from build123d import *

# Parameters (mm, degrees)
SKETCH2_R           = 2.5
BOSS_EXTRUDE1_DEPTH = 10
BOSS_EXTRUDE2_DEPTH = 2
FILLET1_R           = 2


with BuildPart() as part:
    # Sketch2 → Boss-Extrude1 (new body)
    with BuildSketch(Plane(origin=(0, 0, 0), x_dir=(1, 0, 0), z_dir=(0, 1, 0))):
        with BuildLine():
            Line((-68.25, 22.5), (-68.25, -7.5))
            Line((-68.25, -7.5), (-61.75, -7.5))
            Line((-61.75, -7.5), (-61.75, 2.5))
            ThreePointArc((-61.75, 2.5), (-61.164213562, 3.914213562), (-59.75, 4.5))
            Line((-59.75, 4.5), (-40.25, 4.5))
            ThreePointArc((-40.25, 4.5), (-38.835786438, 3.914213562), (-38.25, 2.5))
            Line((-38.25, 2.5), (-38.25, -2))
            ThreePointArc((-38.25, -2), (-37.664213562, -3.414213562), (-36.25, -4))
            Line((-36.25, -4), (1.75, -4))
            ThreePointArc((1.75, -4), (3.164213562, -3.414213562), (3.75, -2))
            Line((3.75, -2), (3.75, 2.5))
            ThreePointArc((3.75, 2.5), (4.335786438, 3.914213562), (5.75, 4.5))
            Line((5.75, 4.5), (25.25, 4.5))
            ThreePointArc((25.25, 4.5), (26.664213562, 3.914213562), (27.25, 2.5))
            Line((27.25, 2.5), (27.25, -7.5))
            Line((27.25, -7.5), (33.75, -7.5))
            Line((33.75, -7.5), (33.75, 22.5))
            Line((33.75, 22.5), (27.25, 22.5))
            Line((27.25, 22.5), (27.25, 12.5))
            ThreePointArc((27.25, 12.5), (26.664213562, 11.085786438), (25.25, 10.5))
            Line((25.25, 10.5), (5.75, 10.5))
            ThreePointArc((5.75, 10.5), (4.335786438, 11.085786438), (3.75, 12.5))
            Line((3.75, 12.5), (3.75, 17))
            ThreePointArc((3.75, 17), (3.164213562, 18.414213562), (1.75, 19))
            Line((1.75, 19), (-36.25, 19))
            ThreePointArc((-36.25, 19), (-37.664213562, 18.414213562), (-38.25, 17))
            Line((-38.25, 17), (-38.25, 12.5))
            ThreePointArc((-38.25, 12.5), (-38.835786438, 11.085786438), (-40.25, 10.5))
            Line((-40.25, 10.5), (-59.75, 10.5))
            ThreePointArc((-59.75, 10.5), (-61.164213562, 11.085786438), (-61.75, 12.5))
            Line((-61.75, 12.5), (-61.75, 22.5))
            Line((-61.75, 22.5), (-68.25, 22.5))
        make_face()
        with Locations((-34.5, 0)):
            Circle(SKETCH2_R, mode=Mode.SUBTRACT)
        Circle(SKETCH2_R, mode=Mode.SUBTRACT)
        with Locations((-34.5, 15)):
            Circle(SKETCH2_R, mode=Mode.SUBTRACT)
        with Locations((0, 15)):
            Circle(SKETCH2_R, mode=Mode.SUBTRACT)
        with Locations((30.25, 19)):
            Circle(SKETCH2_R, mode=Mode.SUBTRACT)
        with Locations((30.25, -4)):
            Circle(SKETCH2_R, mode=Mode.SUBTRACT)
        with Locations((-64.75, -4)):
            Circle(SKETCH2_R, mode=Mode.SUBTRACT)
        with Locations((-64.75, 19)):
            Circle(SKETCH2_R, mode=Mode.SUBTRACT)
    extrude(amount=-BOSS_EXTRUDE1_DEPTH)

    # Sketch3 → Boss-Extrude2 (add)
    with BuildSketch(Plane(origin=(0, 0, 0), x_dir=(1, 0, 0), z_dir=(0, 1, 0))):
        with BuildLine():
            Line((-35.95, 11.814485913), (-35.95, 3.185514087))
            ThreePointArc((-35.95, 3.185514087), (-34.5, 3.5), (-33.05, 3.185514087))
            Line((-33.05, 3.185514087), (-33.05, 11.814485913))
            ThreePointArc((-33.05, 11.814485913), (-34.5, 11.5), (-35.95, 11.814485913))
        make_face()
        with BuildLine():
            ThreePointArc((-1.45, 3.185514087), (0, 3.5), (1.45, 3.185514087))
            Line((1.45, 3.185514087), (1.45, 11.814485913))
            ThreePointArc((1.45, 11.814485913), (0, 11.5), (-1.45, 11.814485913))
            Line((-1.45, 11.814485913), (-1.45, 3.185514087))
        make_face()
    extrude(amount=BOSS_EXTRUDE2_DEPTH)

    # Fillet1
    fillet1_edges = [part.edges().sort_by_distance(p)[0] for p in [
        (27.25, -5, -22.5),
        (33.75, -5, -22.5),
        (33.75, -5, 7.5),
        (27.25, -5, 7.5),
        (-61.75, -5, 7.5),
        (-68.25, -5, 7.5),
        (-68.25, -5, -22.5),
        (-61.75, -5, -22.5),
    ]]
    fillet(fillet1_edges, radius=FILLET1_R)


solid = part.part
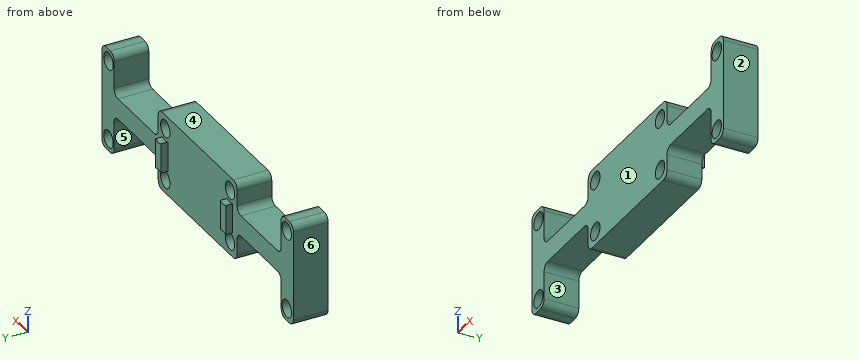
CAD build for the part. Positions are in the model's coordinates, mm. Face numbers are marked on the shaded views. A direction names the side the tool comes from. Give positions to 0.01 mm unless a question says otherwise; leave off trailing zeros. Loops run counter-clockwise (first coordinate to the right, second up) from the corner with the lowest first, then second, coordinate; pieces in that order, holes last. Notation, with made-up numbers: M 55.5,76.25 L 61.5,76.25 A35 ccw 61.5,114.25 Z; hole C 59.5,4 d8. An arc over 180 degrees is marked long. One line per question, with ' | ' between items. Start each with the question number.
1. Saw through at A-A on z = 0. Give the cut face in (x, y).
2. 3-axis set-ups, long thin cutter, end or side, ignore diameter. For the marked faces 4, 5 and 6: which of +Z, -Z, +X, -X, +Y, -Y reach the whole face in a straight line?
3. Saw through at C-C on y = -5.25. State how many separate pieces and enclosed holes the cut face has, plus the area to 3 significant figures.
4. Saw through at D-D on x = 0. Give the cut face in (y, z).
5. Flat gauge pins, fed straight in: pin 1 (6.5 mm diameter, centred on x = -64.75, z = -19, fed in from +Y); pin 2 (1.6 mm diameter, centred on y = 1.5, z = -9, fed in from +X); pin 3 (4.5 mm diameter, centred on x = 0, z = -15, fed in from +Y); pin 4 (1 mm diameter, centred on x = -49.5, y = -5, fed in from -Z). Where does each tip first touch, or does it go through?
6. Saw through at B-B on x = 30.25. Give the cut face in (y, z), plus the area to 3 significant figures.
7. Probe L1, parallel to Z at x = 0, y = -4; L2, parallel to X at y = -7, z = 0; L3, parallel to Z at x = -64.75, y = -7.5. List the from-to ranges inside material, lowest first. Write a range as from..to.
8. Two-plate mould, pull along X, no slides. Class the marked faces 1, 2 and 3: pulls with the +X half, pulls with the -X half, needs draft (parallel to the pull), parting line crosses it, or undercut.
Result sheet:
1) outline: M -68.25,-10 L -61.75,-10 L -61.75,0 L -68.25,0 Z; M -38.25,-10 L -37,-10 L -37,0 L -38.25,0 Z; M -32,-10 L -2.5,-10 L -2.5,0 L -32,0 Z; M 2.5,-10 L 3.75,-10 L 3.75,0 L 2.5,0 Z; M 27.25,-10 L 33.75,-10 L 33.75,0 L 27.25,0 Z
2) face 4: +Z, +Y, -Y | face 5: -Z, +Y, -Y | face 6: +Z, -Z, -X, +Y, -Y
3) separate pieces: 1 | enclosed holes: 8 | area: 1,480 mm^2
4) outline: M -10,-19 L 0,-19 L 0,-17.5 L -10,-17.5 Z; M -10,-12.5 L 0,-12.5 L 0,-11.5 L 2,-11.5 L 2,-3.5 L 0,-3.5 L 0,-2.5 L -10,-2.5 Z; M -10,2.5 L 0,2.5 L 0,4 L -10,4 Z
5) pin 1: stops at y = 0 | pin 2: stops at x = 1.45 | pin 3: passes through | pin 4: stops at z = -10.5
6) outline: M -10,-22.5 L 0,-22.5 L 0,-21.5 L -10,-21.5 Z; M -10,-16.5 L 0,-16.5 L 0,1.5 L -10,1.5 Z; M -10,6.5 L 0,6.5 L 0,7.5 L -10,7.5 Z | area: 200 mm^2
7) L1: z = -19..-17.5, -12.5..-2.5, 2.5..4 | L2: x = -68.25..-61.75, -38.25..-37, -32..-2.5, 2.5..3.75, 27.25..33.75 | L3: z = -22.5..-21.5, -16.5..1.5, 6.5..7.5
8) face 1: needs draft | face 2: pulls with the +X half | face 3: undercut
